CAD build for the part. Positions are in the model's coordinates, mm. Round coordinates to 2 decimals unless told otherwise and drop trailing zeros. Order: outer loops, then holes, each group sorted by start corner. A loop starts at its lowest first (then second) coordinate and runs counter-clockwise, first axis right, second up. Notation, with made-up numbers: (45, 73) - (75, 73) arc R19 cw to (75, 103) - close; hole circle Ø7 at (32, -5.75). An arc over 180 degrees is marked (long way). Write item = value, one per line.
from build123d import *

# Parameters (mm, degrees)
BOSS_EXTRUDE1_DEPTH = 45
SKETCH2_R           = 3
CUT_EXTRUDE1_DEPTH  = 46
CUT_EXTRUDE3_DEPTH  = 46


with BuildPart() as part:
    # Sketch1 → Boss-Extrude1 (new body)
    with BuildSketch(Plane(origin=(0, 0, 0), x_dir=(1, 0, 0), z_dir=(0, 1, 0))):
        with BuildLine():
            Line((-33.134005589, -22.163352058), (76.865994411, -22.163352058))
            Line((76.865994411, -22.163352058), (76.865994411, -2.163352058))
            Line((76.865994411, -2.163352058), (62.388671822, 22.912106224))
            ThreePointArc((62.388671822, 22.912106224), (21.865994411, 7.836647942), (-18.656683, 22.912106224))
            Line((-18.656683, 22.912106224), (-33.134005589, -2.163352058))
            Line((-33.134005589, -2.163352058), (-33.134005589, -22.163352058))
        make_face()
    extrude(amount=BOSS_EXTRUDE1_DEPTH)

    # Sketch2 → Cut-Extrude1 (cut, through all)
    with BuildSketch(Plane(origin=(0, 45, 0), x_dir=(1, 0, 0), z_dir=(0, 1, 0))):
        with Locations((-23.134005589, -7.163352058)):
            Circle(SKETCH2_R)
        with Locations((66.865994411, -7.163352058)):
            Circle(SKETCH2_R)
    extrude(amount=-CUT_EXTRUDE1_DEPTH, mode=Mode.SUBTRACT)

    # Sketch3 → Cut-Extrude3 (cut, through all)
    with BuildSketch(Plane.XZ):
        Polygon((-12.082515606, -24.049109598), (-33.134005589, 2.163352058), (-36.114163106, -37.146188521), align=None)
        Polygon((79.846151928, -37.146188521), (55.814504429, -24.049109598), (76.865994411, 2.163352058), align=None)
    extrude(amount=-CUT_EXTRUDE3_DEPTH, mode=Mode.SUBTRACT)


solid = part.part
(1) Pull direction X, two halves, no side cores. Call faces 1 (the flat face through (21, 22, 22.163)), 2 (the cylindrical face through (-26.13, 22.82, 7.03)), 3 (the flat face through (-33.134, 22, 12)): released by +X, released by -X, zero draft, split by the parting line, or undercut.
Solved:
face_1 = zero draft
face_2 = undercut
face_3 = released by -X
(2) Band-saw the part on B-B on y = 10.5. List the corners of the cut face in (x, z), plus the area to 3 significant figures.
Solved:
outline = (-33.13, 2.16) - (-15.22, -20.15) arc R62 cw to (58.95, -20.15) - (76.87, 2.16) - (76.87, 22.16) - (-33.13, 22.16) - close; hole circle Ø6 at (-23.13, 7.16); hole circle Ø6 at (66.87, 7.16)
area = 3,580 mm²
(3) Band-saw the part on A-A on z = -14. List the corners of the cut face in (x, y).
Solved:
outline = (-20.15, 0) - (-5.08, 0) - (-5.08, 45) - (-20.15, 45) - close; (48.82, 0) - (63.89, 0) - (63.89, 45) - (48.82, 45) - close
(4) Band-saw the part on C-C on x = 65. List the corners of the cut face in (y, z).
Solved:
outline = (0, -12.61) - (45, -12.61) - (45, 4.81) - (0, 4.81) - close; (0, 9.51) - (45, 9.51) - (45, 22.16) - (0, 22.16) - close
(5) Drop flat-ended pins along their axis: pin 1 (5.5 mm diameter, centred on x = 66.87, z = 7.16, fed in from -Y); pin 2 (9.5 mm diameter, centred on x = -23.13, z = 7.16, fed in from +Y); pin 3 (4 mm diameter, centred on x = 38.5, y = 39.5, fed in from -Z); pin 4 (2 mm diameter, centred on y = 9, z = -3, fed in from +X). Give the stop position or say it passes through.
Solved:
pin_1 = through
pin_2 = 45
pin_3 = -10.7
pin_4 = 73.52
(6) Band-saw the part on D-D on z = -2.5. List the corners of the cut face in (x, y), plus the area to 3 significant figures.
Solved:
outline = (-29.39, 0) - (73.12, 0) - (73.12, 45) - (-29.39, 45) - close
area = 4,610 mm²
(7) Probe line 1 along X through (y, z) = (32, 5); line 2 along Z through (x, y) = (69.5, 39); line 3 along Z through (x, y) = (67.5, 36.5). List the from-to ranges inside material, lowest first.
Solved:
line_1 = -33.13 to -25.21, -21.06 to 64.79, 68.94 to 76.87
line_2 = -7.01 to 5.73, 8.6 to 22.16
line_3 = -9.5 to 4.23, 10.1 to 22.16
